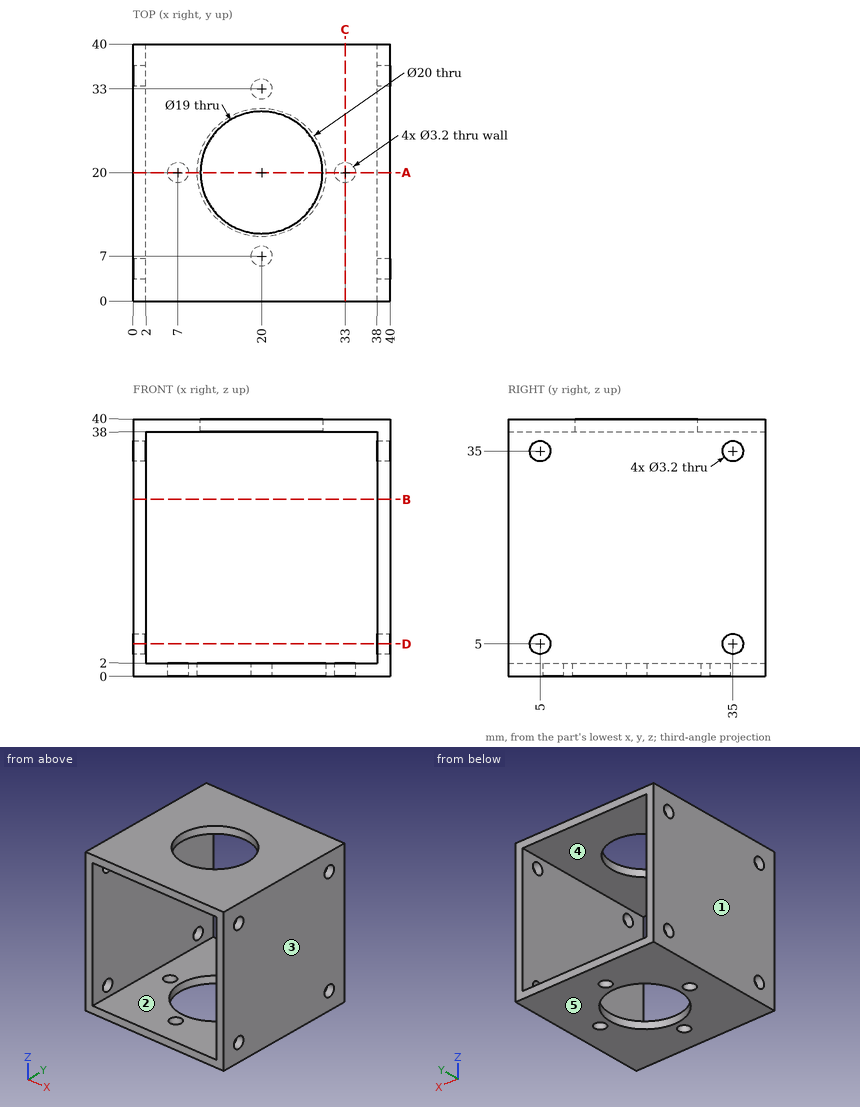
Can you work these out from the drawing? Everything is in mm from the part's minimum corner. A direction names the side the tool comes from. Round coordinates to 2 decimals unless told otherwise and drop trailing zeros. Order: outer loops, then holes, each group sorted by start corner. A loop starts at its lowest first (then second) coordinate and runs counter-clockwise, first axis right, second up. Notation, with made-up numbers: M 4.5,74 L 62.5,74 A19 ccw 62.5,89 Z; hole C 40,44.5 d8. An arc over 180 degrees is marked long. One line per question, with ' | ' between items.
1) If we mould it in two halves opening along X, with no side actions, what happens to the marked faces 1, 2 and 3? For each: +X half, -X half, draft (parallel to the pull), parting line (faces both ways), or undercut.
Working result:
face 1: -X half | face 2: undercut | face 3: +X half
2) For the marked faces 4 and 5, which set-ups out of +Z, -Z, +X, -X, +Y, -Y let a thin tool reach every point of the face, with its end or its side?
Working result:
face 4: +Y, -Y | face 5: -Z, +X, -X, +Y, -Y
3) I want a section at D-D, the plane z = 5. Write out the boundary of the cut face in (x, y), then the cut area to 3 significant figures.
Working result:
outline: M 0,0 L 2,0 L 2,3.4 L 0,3.4 Z; M 0,6.6 L 2,6.6 L 2,33.4 L 0,33.4 Z; M 0,36.6 L 2,36.6 L 2,40 L 0,40 Z; M 38,0 L 40,0 L 40,3.4 L 38,3.4 Z; M 38,6.6 L 40,6.6 L 40,33.4 L 38,33.4 Z; M 38,36.6 L 40,36.6 L 40,40 L 38,40 Z | area: 134 mm²
4) I want a section at C-C, the plane x = 33. Write out the boundary of the cut face in (y, z), then the cut area to 3 significant figures.
Working result:
outline: M 0,0 L 18.4,0 L 18.4,2 L 0,2 Z; M 0,38 L 40,38 L 40,40 L 0,40 Z; M 21.6,0 L 40,0 L 40,2 L 21.6,2 Z | area: 154 mm²
5) I want a section at B-B, the plane z = 27.5. Write out the boundary of the cut face in (x, y).
Working result:
outline: M 0,0 L 2,0 L 2,40 L 0,40 Z; M 38,0 L 40,0 L 40,40 L 38,40 Z
6) I need wall thicknesses on line 1 along Y through (x, z) = (20, 1.15); line 2 along X through (y, z) = (12.5, 28.5). Which ranges of each line are inside material? Lowest first, please.
Working result:
line 1: 0 to 5.4, 8.6 to 10, 30 to 31.4, 34.6 to 40 | line 2: 0 to 2, 38 to 40
7) I want a section at A-A, the plane y = 20. Write out the boundary of the cut face in (x, z).
Working result:
outline: M 0,0 L 5.4,0 L 5.4,2 L 2,2 L 2,38 L 10.5,38 L 10.5,40 L 0,40 Z; M 8.6,0 L 10,0 L 10,2 L 8.6,2 Z; M 29.5,38 L 38,38 L 38,2 L 34.6,2 L 34.6,0 L 40,0 L 40,40 L 29.5,40 Z; M 30,0 L 31.4,0 L 31.4,2 L 30,2 Z
